The listing builds one solid part. Answer for the finished solid, in the listing's coordinates (mm). A direction names the side the tool comes from. Coordinates: 2 decimals unless noted, no trailing zeros. Order: outer loops, then holes, each group sorted by start corner. A loop starts at its lowest first (then second) coordinate and runs counter-clockwise, first axis right, second up.
from build123d import *

# Parameters (mm, degrees)
SKETCH1_R           = 1.65
SKETCH1_R_2         = 1.9
SKETCH1_R_3         = 6
BOSS_EXTRUDE1_DEPTH = 5


with BuildPart() as part:
    # Sketch1 → Boss-Extrude1 (new body)
    with BuildSketch(Plane.YZ):
        with BuildLine():
            Line((0, 0), (94.5, 0))
            ThreePointArc((94.5, 0), (97.328427125, 1.171572875), (98.5, 4))
            Line((98.5, 4), (98.5, 60.5))
            ThreePointArc((98.5, 60.5), (97.328427125, 63.328427125), (94.5, 64.5))
            Line((94.5, 64.5), (32.5, 64.5))
            ThreePointArc((32.5, 64.5), (29.671572875, 63.328427125), (28.5, 60.5))
            Line((28.5, 60.5), (28.5, 46))
            ThreePointArc((28.5, 46), (27.328427125, 43.171572875), (24.5, 42))
            Line((24.5, 42), (0, 42))
            ThreePointArc((0, 42), (-21, 21), (0, 0))
        make_face()
        with Locations(Location((-15.5, 21, 0), (0, 0, 270))):
            Circle(SKETCH1_R, mode=Mode.SUBTRACT)
        with Locations(Location((49.5, 21, 0), (0, 0, 270))):
            Circle(SKETCH1_R_2, mode=Mode.SUBTRACT)
        with Locations(Location((65, 14, 0), (0, 0, 270))):
            Circle(SKETCH1_R_3, mode=Mode.SUBTRACT)
        with Locations(Location((57.25, 34.423393759, 0), (0, 0, 270))):
            Circle(SKETCH1_R_2, mode=Mode.SUBTRACT)
        with Locations(Location((72.75, 34.423393759, 0), (0, 0, 270))):
            Circle(SKETCH1_R_2, mode=Mode.SUBTRACT)
        with Locations(Location((80.5, 21, 0), (0, 0, 270))):
            Circle(SKETCH1_R_2, mode=Mode.SUBTRACT)
        with Locations(Location((72.75, 7.576606241, 0), (0, 0, 270))):
            Circle(SKETCH1_R_2, mode=Mode.SUBTRACT)
        with Locations(Location((57.25, 7.576606241, 0), (0, 0, 270))):
            Circle(SKETCH1_R_2, mode=Mode.SUBTRACT)
        with Locations(Location((0, 36.5, 0), (0, 0, 270))):
            Circle(SKETCH1_R, mode=Mode.SUBTRACT)
        with Locations(Location((15.5, 21, 0), (0, 0, 270))):
            Circle(SKETCH1_R, mode=Mode.SUBTRACT)
        with Locations(Location((0, 5.5, 0), (0, 0, 270))):
            Circle(SKETCH1_R, mode=Mode.SUBTRACT)
    extrude(amount=BOSS_EXTRUDE1_DEPTH)


solid = part.part
1) Determine the mould class of faces 1 (the face through (0, 51, 33)), 2 (the face through (2, 98.5, 32)), 3 (the face through (2.465, 55.395, 34.835)) for opening direction Y: released by +Y, released by -Y, zero draft, split by the parting line, or undercut.
2) Consider L1, parallel to Y at x = 1.7, z = 21; L2, parallel to Z at x = 4.7, y = 58; L3, parallel to Y at x = 1.7, z = 6. Determine where each line is inside the solid, lowest interval first.
3) Section B-B (x = 1) is taken. Give the number of separate pieces and of enclosed holes in the cut face, then the cut area to 3 significant figures.
4) Section D-D (z = 14) is taken. Give the vertices of the cut face in (x, y), then the cut area to 3 significant figures.
5) A tool of negligible diameter and unlimited length cuts with its end or side. For faces 4 (the face through (2.465, 55.395, 7.988)), 5 (the face through (2, 28.5, 53)), from which of +Z, -Z, +X, -X, +Y, -Y can it reach the whole face along a straight path? Write none if from no direction.
6) Section C-C (y = 15.5) is taken. Give the vertices of the cut face in (x, z), then the cut area to 4 significant figures.
7) Section A-A (y = 72.75) is taken. Give the vertices of the cut face in (x, z), then the cut area to 4 significant figures.
8) Each of these flat-tipped pins is pushed along its axis until it touches: P1, Ø2.5, axis at x = 1.5, y = 18, coming from the +Z side; P2, Ø3, axis at x = 4, z = 23, coming from the -Y side; P3, Ø1.5, axis at x = 2, z = 53, coming from the -Y side. Where does it stop, or does it pass through?
Filled sheet:
1. face 1: zero draft
1. face 2: released by +Y
1. face 3: undercut
2. L1: y = -21 to -17.15, -13.85 to 13.85, 17.15 to 47.6, 51.4 to 78.6, 82.4 to 98.5
2. L2: z = 0 to 5.83, 9.32 to 32.68, 36.17 to 64.5
2. L3: y = -14.7 to -1.57, 1.57 to 56.19, 58.31 to 71.69, 73.81 to 98.5
3. separate pieces: 1
3. enclosed holes: 11
3. area: 6,180 mm2
4. outline: (0, -19.8) - (5, -19.8) - (5, 59) - (0, 59) - close; (0, 71) - (5, 71) - (5, 98.5) - (0, 98.5) - close
4. area: 531 mm2
5. face 4: +X, -X
5. face 5: +Z, +X, -X, -Y
6. outline: (0, 0) - (5, 0) - (5, 19.35) - (0, 19.35) - close; (0, 22.65) - (5, 22.65) - (5, 42) - (0, 42) - close
6. area: 193.5 mm2
7. outline: (0, 0) - (5, 0) - (5, 5.68) - (0, 5.68) - close; (0, 9.48) - (5, 9.48) - (5, 32.52) - (0, 32.52) - close; (0, 36.32) - (5, 36.32) - (5, 64.5) - (0, 64.5) - close
7. area: 284.5 mm2
8. P1: stops at z = 42
8. P2: stops at y = -20.99
8. P3: stops at y = 28.5
